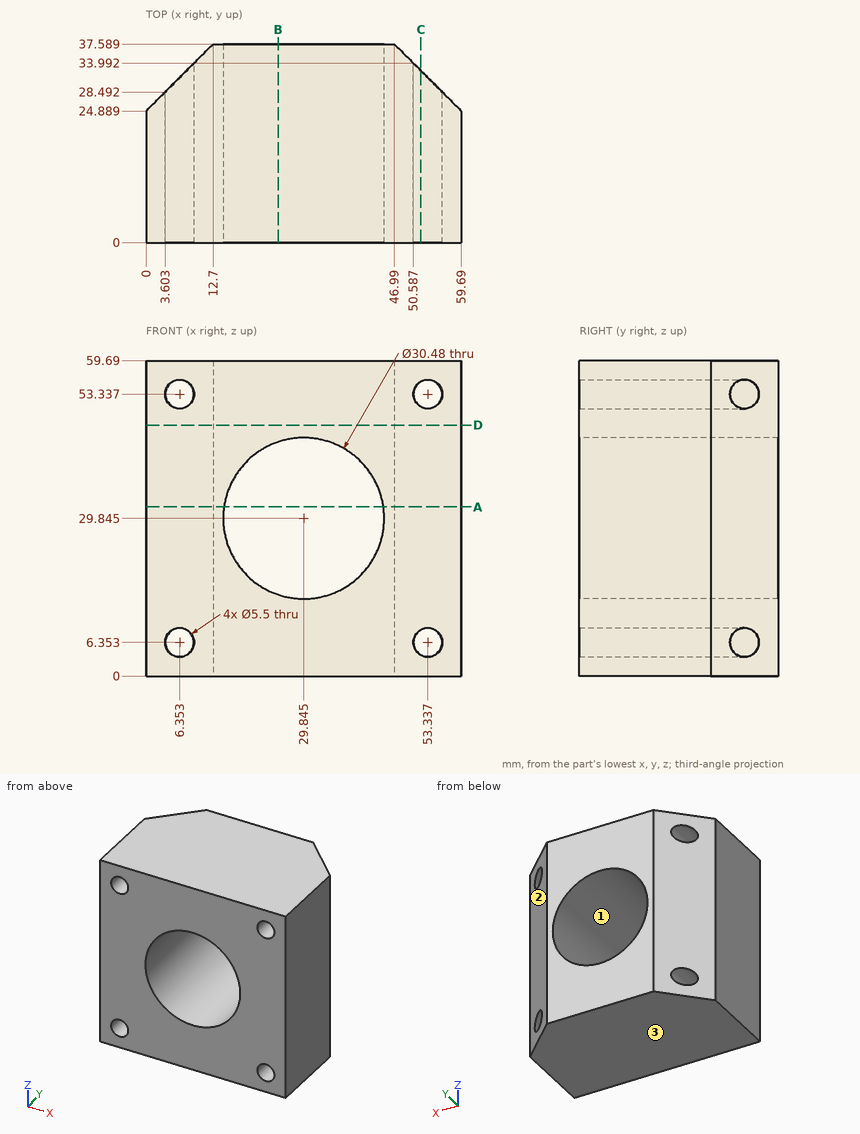
Here's the drawing with two shaded views (mm, measured from the low corner). I have some questions. Give positions to 0.01 mm unless a question says otherwise; leave off trailing zeros. Loops run counter-clockwise (first coordinate to the right, second up) from the corner with the lowest first, then second, coordinate; pieces in that order, holes last. Notation, with made-up numbers: (65, 40.25) -> (96, 40.25) arc R14 cw to (96, 45.25) -> close; hole circle Ø1 at (76, -40). An arc over 180 degrees is marked (long way). One line per item, written item: value.
Q1. We'd pull the mould along Z, two halves only. Please class the marked faces 1, 2 and 3: pulls with the +Z half, pulls with the -Z half, needs draft (parallel to the pull), parting line crosses it, or undercut.
Answers follow:
face 1: undercut
face 2: needs draft
face 3: pulls with the -Z half
Q2. Suppose I cut it at B-B on x = 25. Please give me the cut outline in (y, z) (1 decimal), then the cut area to 3 significant figures.
Answers follow:
outline: (0, 0) -> (37.6, 0) -> (37.6, 15.4) -> (0, 15.4) -> close; (0, 44.3) -> (37.6, 44.3) -> (37.6, 59.7) -> (0, 59.7) -> close
area: 1,160 mm^2
Q3. Suppose I cut it at C-C on x = 52. State how many separate pieces and enclosed holes the cut face has, then the cut area to 3 significant figures.
Answers follow:
separate pieces: 3
enclosed holes: 0
area: 1,630 mm^2
Q4. If I drill on line 1 along Z through (x, y) = (52.5, 8.5); line 2 along Z through (x, y) = (43, 6); line 3 along Z through (x, y) = (27.5, 35.5), over which ranges is the centre line in solid material (lowest first)?
Answers follow:
line 1: 0 to 3.73, 8.97 to 50.72, 55.96 to 59.69
line 2: 0 to 22.15, 37.54 to 59.69
line 3: 0 to 14.79, 44.9 to 59.69
Q5. Suppose I cut it at A-A on z = 32. Please give me the cut outline in (x, y), then the cut area to 3 significant figures.
Answers follow:
outline: (0, 0) -> (14.76, 0) -> (14.76, 37.59) -> (12.7, 37.59) -> (0, 24.89) -> close; (44.93, 0) -> (59.69, 0) -> (59.69, 24.89) -> (46.99, 37.59) -> (44.93, 37.59) -> close
area: 948 mm^2
Q6. I'm going to push a flat-ended pin straight in: pin 1 Ø3.5 at (x, z) = (53.34, 53.34) entering from -Y. Where does the tip first touch, or does it pass through?
Answers follow:
pin 1: through
Q7. Suppose I cut it at D-D on z = 47.5. Please give me the cut outline in (x, y), then the cut area to 3 significant figures.
Answers follow:
outline: (0, 0) -> (59.69, 0) -> (59.69, 24.89) -> (46.99, 37.59) -> (12.7, 37.59) -> (0, 24.89) -> close
area: 2,080 mm^2
